For this review, take the finished solid that the model builds, in its own axes (mm). Give positions to 0.01 mm unless a question says otherwise; leave off trailing zeros. Loops run counter-clockwise (first coordinate to the right, second up) from the corner with the lowest first, then second, coordinate; pieces in that order, holes last.
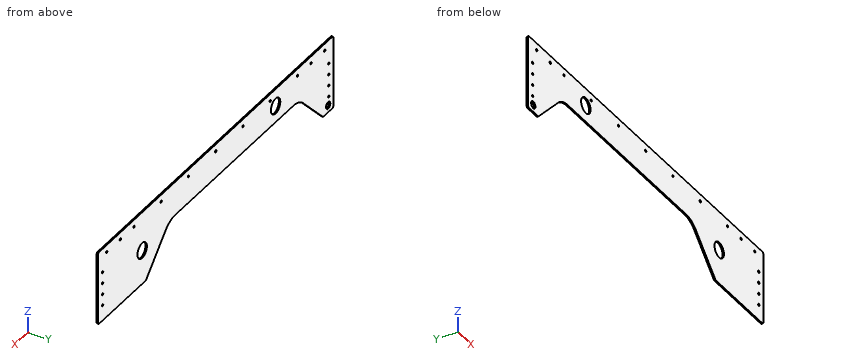
```python
from build123d import *

# Parameters (mm, degrees)
SKETCH1_R           = 17.4625
SKETCH1_R_2         = 2.4257
SKETCH1_R_3         = 7.9375
BOSS_EXTRUDE1_DEPTH = 3.175
FILLET1_R           = 50.8
FILLET2_R           = 3.175


with BuildPart() as part:
    # Sketch1 → Boss-Extrude1 (new body)
    with BuildSketch(Plane(origin=(0, 0, 0), x_dir=(1, 0, 0), z_dir=(0, 1, 0))):
        Polygon((0, 0), (876.3, 0), (876.3, 165.1), (698.5, 165.1), (609.6, 76.2), (127, 76.2), (38.1, 165.1), (0, 165.1), align=None)
        with Locations(Location((214.9475, 38.9255, 0), (0, 0, 270))):
            Circle(SKETCH1_R, mode=Mode.SUBTRACT)
        with Locations(Location((712.16774, 87.9475, 0), (0, 0, 270))):
            Circle(SKETCH1_R, mode=Mode.SUBTRACT)
        with Locations(Location((438.15, 15.875, 0), (0, 0, 270))):
            Circle(SKETCH1_R_2, mode=Mode.SUBTRACT)
        with Locations(Location((539.75, 15.875, 0), (0, 0, 270))):
            Circle(SKETCH1_R_2, mode=Mode.SUBTRACT)
        with Locations(Location((641.35, 15.875, 0), (0, 0, 270))):
            Circle(SKETCH1_R_2, mode=Mode.SUBTRACT)
        with Locations(Location((742.95, 15.875, 0), (0, 0, 270))):
            Circle(SKETCH1_R_2, mode=Mode.SUBTRACT)
        with Locations(Location((844.55, 15.875, 0), (0, 0, 270))):
            Circle(SKETCH1_R_2, mode=Mode.SUBTRACT)
        with Locations(Location((31.75, 15.875, 0), (0, 0, 270))):
            Circle(SKETCH1_R_2, mode=Mode.SUBTRACT)
        with Locations(Location((133.35, 15.875, 0), (0, 0, 270))):
            Circle(SKETCH1_R_2, mode=Mode.SUBTRACT)
        with Locations(Location((234.95, 15.875, 0), (0, 0, 270))):
            Circle(SKETCH1_R_2, mode=Mode.SUBTRACT)
        with Locations(Location((336.55, 15.875, 0), (0, 0, 270))):
            Circle(SKETCH1_R_2, mode=Mode.SUBTRACT)
        with Locations(Location((16.637, 53.975, 0), (0, 0, 270))):
            Circle(SKETCH1_R_2, mode=Mode.SUBTRACT)
        with Locations(Location((16.637, 79.375, 0), (0, 0, 270))):
            Circle(SKETCH1_R_2, mode=Mode.SUBTRACT)
        with Locations(Location((16.637, 104.775, 0), (0, 0, 270))):
            Circle(SKETCH1_R_2, mode=Mode.SUBTRACT)
        with Locations(Location((16.637, 130.175, 0), (0, 0, 270))):
            Circle(SKETCH1_R_2, mode=Mode.SUBTRACT)
        with Locations(Location((859.663, 53.975, 0), (0, 0, 270))):
            Circle(SKETCH1_R_2, mode=Mode.SUBTRACT)
        with Locations(Location((859.663, 79.375, 0), (0, 0, 270))):
            Circle(SKETCH1_R_2, mode=Mode.SUBTRACT)
        with Locations(Location((859.663, 104.775, 0), (0, 0, 270))):
            Circle(SKETCH1_R_2, mode=Mode.SUBTRACT)
        with Locations(Location((859.663, 130.175, 0), (0, 0, 270))):
            Circle(SKETCH1_R_2, mode=Mode.SUBTRACT)
        with Locations(Location((82.55, 15.875, 0), (0, 0, 270))):
            Circle(SKETCH1_R_2, mode=Mode.SUBTRACT)
        with Locations(Location((793.75, 15.875, 0), (0, 0, 270))):
            Circle(SKETCH1_R_2, mode=Mode.SUBTRACT)
        with Locations(Location((19.05, 149.225, 0), (0, 0, 270))):
            Circle(SKETCH1_R_3, mode=Mode.SUBTRACT)
    extrude(amount=BOSS_EXTRUDE1_DEPTH)

    # Fillet1
    fillet1_edges = [part.edges().sort_by_distance(p)[0] for p in [
        (127, 1.5875, -76.2),
        (609.6, 1.5875, -76.2),
    ]]
    fillet(fillet1_edges, radius=FILLET1_R)

    # Fillet2
    fillet2_edges = [part.edges().sort_by_distance(p)[0] for p in [
        (698.5, 1.5875, -165.1),
        (876.3, 1.5875, -165.1),
        (876.3, 1.5875, 0),
        (0, 1.5875, 0),
        (0, 1.5875, -165.1),
        (38.1, 1.5875, -165.1),
    ]]
    fillet(fillet2_edges, radius=FILLET2_R)


solid = part.part
```
Item 1: Take a section at A-A on z = -33.5. Give the boundary of the cut face in (x, y) (3 decimals).
Answer:
outline: (0, 0) - (198.349, 0) - (198.349, 3.175) - (0, 3.175) - close; (231.546, 0) - (876.3, 0) - (876.3, 3.175) - (231.546, 3.175) - close
Item 2: Clearance check with flat-ended pins moving along their axes: pin 1 Ø4.5 at (x, z) = (844.55, -15.875) entering from +Y; pin 2 Ø5.5 at (x, z) = (31.75, -15.875) entering from -Y. State where each tip first meets the part, or that it passes through.
Answer:
pin 1: passes through
pin 2: stops at y = 0
Item 3: Take a section at D-D on x = 600. Give the boundary of the cut face in (y, z) (3 decimals).
Answer:
outline: (0, -77.505) - (3.175, -77.505) - (3.175, 0) - (0, 0) - close
Item 4: For L1, parallel to Z at x = 439, y = 2.25; L2, parallel to X at y = 0.1, z = -54; L3, parallel to X at y = 0.85, z = -129.5, list the stretches that pass through material, from the lowest coordinate up.
Answer:
L1: z = -76.2 to -18.15, -13.6 to 0
L2: x = 0 to 14.21, 19.06 to 206.13, 223.76 to 857.24, 862.09 to 876.3
L3: x = 0 to 14.31, 18.97 to 73.7, 662.9 to 857.33, 861.99 to 876.3
Item 5: Take a section at C-C on y = 1.55. State how many separate pieces and enclosed holes the cut face has, and give its area (3 significant figures).
Answer:
separate pieces: 1
enclosed holes: 22
area: 91,500 mm2
Item 6: Take a section at B-B on x = 404.5. Give the boundary of the cut face in (y, z) (3 decimals).
Answer:
outline: (0, -76.2) - (3.175, -76.2) - (3.175, 0) - (0, 0) - close
